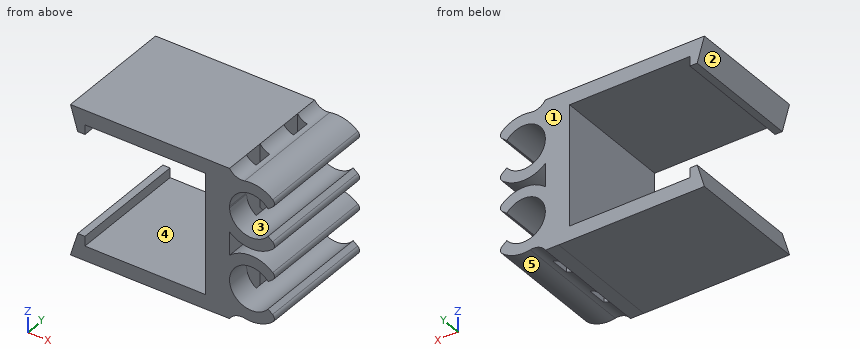
```python
from build123d import *

# Parameters (mm, degrees)
EXTRUDE_1_DEPTH      = 25
CUT_EXTRUDE_4_DEPTH  = 80.457942189
SKETCH_7_W           = 16.60831278
SKETCH_7_H           = 38.473598513
CUT_EXTRUDE_14_DEPTH = 80.457942189
SKETCH_8_W           = 5
SKETCH_8_H           = 30.968526609
EXTRUDE_2_DEPTH      = 25
EXTRUDE_3_DEPTH      = 25
FILLET_2_R           = 3
FILLET_4_R           = 1
SKETCH_10_W          = 2
SKETCH_10_H          = 4
CUT_EXTRUDE_15_DEPTH = 78.792556685


with BuildPart() as part:
    # Эскиз1 → Бобышка-Вытянуть1 (new body)
    with BuildSketch(Plane(origin=(0, 0, 0), x_dir=(1, 0, 0), z_dir=(0, 1, 0))):
        Polygon((-66.825757576, 34.969739794), (-66.825757576, 29.969739794), (-63.825757576, 29.969739794), (-63.825757576, 31.969739794), (-38.825757576, 31.969739794), (-38.825757576, 6.969739794), (-63.825757576, 6.969739794), (-63.825757576, 8.969739794), (-66.825757576, 8.969739794), (-66.825757576, 3.969739794), (-22.123470102, 3.969739794), (-36.579007505, 34.969739794), align=None)
    extrude(amount=EXTRUDE_1_DEPTH)

    # Эскиз3 → Вырез-Вытянуть4 (cut, through all)
    with BuildSketch(Plane.XZ):
        Polygon((-66.825757576, -3.969739794), (-65.325757576, -8.969739794), (-66.825757576, -8.969739794), align=None)
        Polygon((-66.825757576, -29.969739794), (-66.825757576, -34.969739794), (-65.325757576, -29.969739794), align=None)
    extrude(amount=-CUT_EXTRUDE_4_DEPTH, mode=Mode.SUBTRACT)

    # Эскиз7 → Вырез-Вытянуть14 (cut, through all)
    with BuildSketch(Plane(origin=(0, 0, 0), x_dir=(-1, 0, 0), z_dir=(0, -1, 0))):
        with Locations((27.703474463, 20.539743139)):
            Rectangle(SKETCH_7_W, SKETCH_7_H)
    extrude(amount=-CUT_EXTRUDE_14_DEPTH, mode=Mode.SUBTRACT)

    # Эскиз8 → Бобышка-Вытянуть2 (add)
    with BuildSketch(Plane(origin=(0, 0, 0), x_dir=(-1, 0, 0), z_dir=(0, -1, 0))):
        with Locations((36.298943925, 19.454003098)):
            Rectangle(SKETCH_8_W, SKETCH_8_H)
    extrude(amount=-EXTRUDE_2_DEPTH)

    # Эскиз9 → Бобышка-Вытянуть3 (add)
    with BuildSketch(Plane.XZ):
        with BuildLine():
            Line((-25.798943925, -9.121669553), (-24.000865345, -7.695483003))
            ThreePointArc((-24.000865345, -7.695483003), (-36.096342696, -11.954003099), (-24.000865345, -16.212523195))
            Line((-24.000865345, -16.212523195), (-25.798943925, -14.786336644))
            ThreePointArc((-25.798943925, -14.786336644), (-33.80140029, -11.954003099), (-25.798943925, -9.121669553))
        make_face()
        with BuildLine():
            Line((-25.798943925, -24.130682885), (-24.000865345, -22.7126007))
            ThreePointArc((-24.000865345, -22.7126007), (-36.0856317, -26.954003099), (-24.000865345, -31.195405497))
            Line((-24.000865345, -31.195405497), (-25.798943925, -29.777323313))
            ThreePointArc((-25.798943925, -29.777323313), (-33.795735785, -26.954003099), (-25.798943925, -24.130682885))
        make_face()
    extrude(amount=-EXTRUDE_3_DEPTH)

    # Скругление2
    # the kernel refuses this fillet: 3 mm, written as the material it adds along each edge
    with BuildSketch(Plane(origin=(-33.798943925, 25, -6.859434417), x_dir=(0, 0, 1), z_dir=(0, -1, 0))) as fillet_2_piece_1:
        with BuildLine():
            CenterArc((4.502629254, -2.529514158), FILLET_2_R, 122.523458888, 69.079199353)
            Line((1.563931496, -3.132884263), (1.505157541, -3.144951665))
            ThreePointArc((1.505157541, -3.144951665), (0.933475042, -1.490808901), (-0.044969279, -0.039721077))
            Line((-0.044969279, -0.039721077), (0, 0.06))
            ThreePointArc((0, 0.06), (1.444847312, 0.06), (2.85743593, 0.050590283))
            Line((2.85743593, 0.050590283), (2.889694623, 0))
        make_face()
    extrude(amount=25)
    with BuildSketch(Plane(origin=(-33.798943925, 25, -32.034271886), x_dir=(0, 0, -1), z_dir=(0, -1, 0))) as fillet_2_piece_2:
        with BuildLine():
            CenterArc((4.507255062, 2.535656843), FILLET_2_R, 168.421178081, 69.274223823)
            Line((1.568306542, 3.137804332), (1.509527572, 3.149847282))
            ThreePointArc((1.509527572, 3.149847282), (0.936720457, 1.492647534), (-0.044913828, 0.039783766))
            Line((-0.044913828, 0.039783766), (0, -0.06))
            ThreePointArc((0, -0.06), (1.451997259, -0.06), (2.871929307, -0.050713137))
            Line((2.871929307, -0.050713137), (2.903994517, 0))
        make_face()
    extrude(amount=25)

    # Скругление4
    fillet_4_edges = [part.edges().sort_by_distance(p)[0] for p in [
        (-24.000865345, 12.5, -7.695483003),
        (-24.000865345, 12.5, -16.212523195),
        (-24.000865345, 12.5, -22.7126007),
        (-24.000865345, 12.5, -31.195405497),
    ]]
    fillet(fillet_4_edges, radius=FILLET_4_R)

    # Эскиз10 → Вырез-Вытянуть15 (cut, through all)
    with BuildSketch(Plane.XY.offset(-3.969739794)):
        with Locations((-32.798943925, 18)):
            Rectangle(SKETCH_10_W, SKETCH_10_H)
        with Locations((-32.798943925, 7)):
            Rectangle(SKETCH_10_W, SKETCH_10_H)
    extrude(amount=-CUT_EXTRUDE_15_DEPTH, mode=Mode.SUBTRACT)


solid = part.part
```
For this review, take the finished solid that the model builds, in its own axes (mm). Face numbers are marked on the shaded views. A direction names the side the tool comes from. Round coordinates to 2 decimals unless told otherwise and drop trailing zeros. Write each loop counter-clockwise with the first axis right and the second up, starting at its lowest first coordinate (ties: lowest second). Pieces come first, ordered by that corner, then holes. Notation, with made-up numbers: (3.5, -7.5) - (13.5, -7.5) arc R17 cw to (13.5, -0.5) - close; hole circle Ø1 at (51.5, -5.5). An arc over 180 degrees is marked (long way). Put each result on its own line as item: value.
Q1. We need section B-B (x = -29). Give the boundary of the cut face in (y, z).
Solved:
outline: (0, -33.73) - (25, -33.73) - (25, -31.44) - (0, -31.44) - close; (0, -22.47) - (25, -22.47) - (25, -20.17) - (0, -20.17) - close; (0, -18.74) - (25, -18.74) - (25, -16.45) - (0, -16.45) - close; (0, -7.46) - (25, -7.46) - (25, -5.16) - (0, -5.16) - close
Q2. We need section A-A (x = -45). Give the boundary of the cut face in (y, z), and give its area (3 significant figures).
Solved:
outline: (0, -34.97) - (25, -34.97) - (25, -31.97) - (0, -31.97) - close; (0, -6.97) - (25, -6.97) - (25, -3.97) - (0, -3.97) - close
area: 150 mm2
Q3. Mouldability with a two-part tool opening along X and no side actions: class the marked faces 1, 2 and 3 as released by +X, released by -X, zero draft, split by the parting line, or undercut.
Solved:
face 1: zero draft
face 2: released by -X
face 3: undercut
Q4. Wall thickness on probe 1 along Z at (x, y) = (-27.5, 8.25); probe 2 along Z at (x, y) = (-29, 15.5); probe 3 along Z at (x, y) = (-40, 9.75): over which ranges is each line inside the solid? List them lowest first.
Solved:
probe 1: z = -33.5 to -31.08, -22.83 to -20.41, -18.51 to -16.08, -7.83 to -5.4
probe 2: z = -33.73 to -31.44, -22.47 to -20.17, -18.74 to -16.45, -7.46 to -5.16
probe 3: z = -34.97 to -31.97, -6.97 to -3.97
Q5. We need section C-C (z = -28). Give the boundary of the cut face in (x, y), and give its area (3 significant figures).
Solved:
outline: (-38.83, 0) - (-33.67, 0) - (-33.67, 5) - (-33.8, 5) - (-33.8, 9) - (-33.67, 9) - (-33.67, 16) - (-33.8, 16) - (-33.8, 20) - (-33.67, 20) - (-33.67, 25) - (-38.83, 25) - close
area: 128 mm2
Q6. Machinability: for the marked faces 4 and 5, which of the approach directions +Z, -Z, +X, -X, +Y, -Y give a long, thin tool a straight path to every point of the face, cutting with its end or side? Answer none if there is none.
Solved:
face 4: +Y, -Y
face 5: -Z, +Y, -Y
Q7. Insertion check: pin 1 Ø2 at (x, z) = (-32.5, -27.5) entering from -Y; pin 2 Ø8 at (y, z) = (13, -24.5) entering from +X; pin 3 Ø1 at (x, y) = (-30.5, 5) entering from +Z; pin 4 Ø3 at (y, z) = (7.5, -31.5) entering from -X. Each pin has a flat end and moves straight along its axis. Give the tip position at first contact, or say it passes through.
Solved:
pin 1: passes through
pin 2: stops at x = -24.48
pin 3: stops at z = -5.19
pin 4: stops at x = -66.23
